Read the model definition and answer for the solid it produces. Units are mm, in the model's axes. Face numbers are marked on the shaded views. A direction names the side the tool comes from. Round coordinates to 2 decimals unless told otherwise and drop trailing zeros. Write each loop counter-clockwise with the first axis right and the second up, starting at its lowest first coordinate (ties: lowest second). Pieces come first, ordered by that corner, then holes. Notation, with made-up numbers: (5.5, 71.5) - (50.5, 71.5) arc R13 cw to (50.5, 85.5) - close; hole circle Ø6 at (39, 0.5). An arc over 180 degrees is marked (long way). Answer as CSV lines item,"result". Start each with the question number.
1) Find section A-A on x = 8.75. Determine the outline of the cut face in (y, z), then the cut area to 3 significant figures.
2) Find section B-B on y = 10. Determine the outline of the cut face in (x, z), then the cut area to 4 significant figures.
3) For a pull along Y with two mould halves and no side action, classify the marked faces 5, 6 and 7 as +Y half, -Y half, draft (parallel to the pull), parting line (faces both ways), or undercut.
4) Consider line 1 along Y through (x, z) = (7.5, 2.75); line 2 along X through (y, z) = (3.75, 7); line 3 along Y through (x, z) = (10, 5). Determine where each line is inside the solid, lowest interval first.
5) Each of these flat-tipped pins is pushed along its axis until it touches: pin 1 (4 mm diameter, centred on x = 15, z = 5, fed in from -Y); pin 2 (1.2 mm diameter, centred on x = 21, y = -1.5, fed in from +Z); pin 3 (0.6 mm diameter, centred on x = 13.5, y = 3.5, fed in from -Z). Where does it stop, or does it pass through?
6) Which of the six approach directions +Z, -Z, +X, -X, +Y, -Y give full straight-line access (tool end or side, diameter ignored) to the marked faces 1, 2, 3 and 4?
from build123d import *

# Parameters (mm, degrees)
BOSS_EXTRUDE1_DEPTH = 7.6
SKETCH2_W           = 17
SKETCH2_H           = 8.9
BOSS_EXTRUDE2_DEPTH = 2
SKETCH3_W           = 20
SKETCH3_H           = 2.43
BOSS_EXTRUDE3_DEPTH = 7.4
SKETCH4_W           = 18
SKETCH4_H           = 2.9
BOSS_EXTRUDE4_DEPTH = 7.67
CUT_EXTRUDE1_DEPTH  = 0.95
SKETCH6_W           = 1.35
SKETCH6_H           = 6.05
CUT_EXTRUDE2_DEPTH  = 0.8
CHAMFER1_SIZE       = 0.5
CHAMFER2_SIZE       = 1
CHAMFER3_SIZE       = 1
SKETCH7_W           = 2.8
SKETCH7_H           = 1.6
BOSS_EXTRUDE5_DEPTH = 2.8
SKETCH8_W           = 2.8
SKETCH8_H           = 0.8
BOSS_EXTRUDE6_DEPTH = 2
CUT_EXTRUDE3_DEPTH  = 30.270462928
CHAMFER4_SIZE       = 0.5
SKETCH10_W          = 2
SKETCH10_H          = 7.95
SKETCH10_W_2        = 1
CUT_EXTRUDE4_DEPTH  = 1
CUT_EXTRUDE5_DEPTH  = 1
SKETCH12_W          = 2
SKETCH12_H          = 1.1
CUT_EXTRUDE6_DEPTH  = 1


with BuildPart() as part:
    # Sketch1 → Boss-Extrude1 (new body)
    with BuildSketch(Plane(origin=(0, 0, 0), x_dir=(1, 0, 0), z_dir=(0, 1, 0))):
        Polygon((0, 0), (0, -11), (22.6, -11), (22.6, 0), (19.8, 0), (19.8, -8.9), (2.8, -8.9), (2.8, 0), align=None)
    extrude(amount=BOSS_EXTRUDE1_DEPTH)

    # Sketch2 → Boss-Extrude2 (add)
    with BuildSketch(Plane(origin=(0, 7.6, 0), x_dir=(1, 0, 0), z_dir=(0, 1, 0))):
        with Locations((11.3, -4.45)):
            Rectangle(SKETCH2_W, SKETCH2_H)
    extrude(amount=-BOSS_EXTRUDE2_DEPTH)

    # Sketch3 → Boss-Extrude3 (add)
    with BuildSketch(Plane(origin=(0, 7.6, 0), x_dir=(1, 0, 0), z_dir=(0, 1, 0))):
        with Locations((11.3, -1.215)):
            Rectangle(SKETCH3_W, SKETCH3_H)
    extrude(amount=BOSS_EXTRUDE3_DEPTH)

    # Sketch4 → Boss-Extrude4 (add)
    with BuildSketch(Plane.XY.offset(2.43)):
        with Locations((11.3, 13.55)):
            Rectangle(SKETCH4_W, SKETCH4_H)
    extrude(amount=BOSS_EXTRUDE4_DEPTH)

    # Sketch5 → Cut-Extrude1 (cut)
    with BuildSketch(Plane(origin=(0, 0, 0), x_dir=(-1, 0, 0), z_dir=(0, 0, -1))):
        Polygon((-19.8, 11.5), (-19.8, 5.6), (-2.8, 5.6), (-2.8, 11.5), (-2.4, 11.5), (-2.4, 15), (-20.2, 15), (-20.2, 11.5), align=None)
    extrude(amount=-CUT_EXTRUDE1_DEPTH, mode=Mode.SUBTRACT)

    # Sketch6 → Cut-Extrude2 (cut)
    with BuildSketch(Plane(origin=(0, 15, 0), x_dir=(1, 0, 0), z_dir=(0, 1, 0))):
        with Locations((3.8, -3.975)):
            Rectangle(SKETCH6_W, SKETCH6_H)
        with Locations((6.3, -3.975)):
            Rectangle(SKETCH6_W, SKETCH6_H)
        with Locations((8.8, -3.975)):
            Rectangle(SKETCH6_W, SKETCH6_H)
        with Locations((11.3, -3.975)):
            Rectangle(SKETCH6_W, SKETCH6_H)
        with Locations((13.8, -3.975)):
            Rectangle(SKETCH6_W, SKETCH6_H)
        with Locations((16.3, -3.975)):
            Rectangle(SKETCH6_W, SKETCH6_H)
        with Locations((18.8, -3.975)):
            Rectangle(SKETCH6_W, SKETCH6_H)
    extrude(amount=-CUT_EXTRUDE2_DEPTH, mode=Mode.SUBTRACT)

    # Chamfer1
    chamfer1_edges = [part.edges().sort_by_distance(p)[0] for p in [
        (20.3, 13.55, 10.1),
        (2.3, 13.55, 10.1),
    ]]
    chamfer(chamfer1_edges, length=CHAMFER1_SIZE)

    # Chamfer2
    chamfer2_edges = [part.edges().sort_by_distance(p)[0] for p in [
        (11.3, 15, 10.1),
    ]]
    chamfer(chamfer2_edges, length=CHAMFER2_SIZE)

    # Chamfer3
    chamfer3_edges = [part.edges().sort_by_distance(p)[0] for p in [
        (11.3, 7.6, 11),
    ]]
    chamfer(chamfer3_edges, length=CHAMFER3_SIZE)

    # Sketch7 → Boss-Extrude5 (add)
    with BuildSketch(Plane.XZ):
        with Locations((1.4, 0.8)):
            Rectangle(SKETCH7_W, SKETCH7_H)
        with Locations((21.2, 0.8)):
            Rectangle(SKETCH7_W, SKETCH7_H)
    extrude(amount=BOSS_EXTRUDE5_DEPTH)

    # Sketch8 → Boss-Extrude6 (add)
    with BuildSketch(Plane(origin=(0, 0, 0), x_dir=(-1, 0, 0), z_dir=(0, 0, -1))):
        with Locations((-21.2, -2.4)):
            Rectangle(SKETCH8_W, SKETCH8_H)
        with Locations((-1.4, -2.4)):
            Rectangle(SKETCH8_W, SKETCH8_H)
    extrude(amount=BOSS_EXTRUDE6_DEPTH)

    # Sketch9 → Cut-Extrude3 (cut, through all)
    with BuildSketch(Plane.ZY):
        with BuildLine():
            ThreePointArc((1.6, 0), (2.1, -0.5), (2.6, 0))
            Line((2.6, 0), (1.6, 0))
        make_face()
        with BuildLine():
            Line((1.6, 0), (2.6, 0))
            ThreePointArc((2.6, 0), (2.1, 0.5), (1.6, 0))
        make_face()
    extrude(amount=-CUT_EXTRUDE3_DEPTH, mode=Mode.SUBTRACT)

    # Chamfer4
    chamfer4_edges = [part.edges().sort_by_distance(p)[0] for p in [
        (1.4, -2.8, 1.6),
        (21.2, -2.8, 1.6),
    ]]
    chamfer(chamfer4_edges, length=CHAMFER4_SIZE)

    # Sketch10 → Cut-Extrude4 (cut)
    with BuildSketch(Plane.XZ.offset(-5.6)):
        with Locations((4.31, 4.925)):
            Rectangle(SKETCH10_W, SKETCH10_H)
        with Locations((6.64, 4.925)):
            Rectangle(SKETCH10_W, SKETCH10_H)
        with Locations((8.97, 4.925)):
            Rectangle(SKETCH10_W, SKETCH10_H)
        with Locations((11.8, 4.925)):
            Rectangle(SKETCH10_W_2, SKETCH10_H)
        with Locations((10.8, 4.925)):
            Rectangle(SKETCH10_W_2, SKETCH10_H)
        with Locations((13.63, 4.925)):
            Rectangle(SKETCH10_W, SKETCH10_H)
        with Locations((15.96, 4.925)):
            Rectangle(SKETCH10_W, SKETCH10_H)
        with Locations((18.29, 4.925)):
            Rectangle(SKETCH10_W, SKETCH10_H)
    extrude(amount=-CUT_EXTRUDE4_DEPTH, mode=Mode.SUBTRACT)

    # Sketch11 → Cut-Extrude5 (cut)
    with BuildSketch(Plane(origin=(0, 0, 8.9), x_dir=(-1, 0, 0), z_dir=(0, 0, -1))):
        Polygon((-19.29, 6.6), (-19.29, 5.6), (-19.29, 0), (-17.29, 0), (-17.29, 5.6), (-17.29, 6.6), align=None)
        Polygon((-16.96, 5.6), (-16.96, 0), (-14.96, 0), (-14.96, 5.6), (-14.96, 6.6), (-16.96, 6.6), align=None)
        Polygon((-14.63, 5.6), (-14.63, 0), (-12.63, 0), (-12.63, 5.6), (-12.63, 6.6), (-14.63, 6.6), align=None)
        Polygon((-12.3, 5.6), (-12.3, 0), (-10.3, 0), (-10.3, 5.6), (-10.3, 6.6), (-12.3, 6.6), align=None)
        Polygon((-9.97, 5.6), (-9.97, 0), (-7.97, 0), (-7.97, 5.6), (-7.97, 6.6), (-9.97, 6.6), align=None)
        Polygon((-7.64, 5.6), (-7.64, 0), (-5.64, 0), (-5.64, 5.6), (-5.64, 6.6), (-7.64, 6.6), align=None)
        Polygon((-5.31, 5.6), (-5.31, 0), (-3.31, 0), (-3.31, 5.6), (-3.31, 6.6), (-5.31, 6.6), align=None)
    extrude(amount=-CUT_EXTRUDE5_DEPTH, mode=Mode.SUBTRACT)

    # Sketch12 → Cut-Extrude6 (cut)
    with BuildSketch(Plane.XZ):
        with Locations((4.31, 10.45)):
            Rectangle(SKETCH12_W, SKETCH12_H)
        with Locations((6.64, 10.45)):
            Rectangle(SKETCH12_W, SKETCH12_H)
        with Locations((8.97, 10.45)):
            Rectangle(SKETCH12_W, SKETCH12_H)
        with Locations((11.3, 10.45)):
            Rectangle(SKETCH12_W, SKETCH12_H)
        with Locations((13.63, 10.45)):
            Rectangle(SKETCH12_W, SKETCH12_H)
        with Locations((15.96, 10.45)):
            Rectangle(SKETCH12_W, SKETCH12_H)
        with Locations((18.29, 10.45)):
            Rectangle(SKETCH12_W, SKETCH12_H)
    extrude(amount=-CUT_EXTRUDE6_DEPTH, mode=Mode.SUBTRACT)


solid = part.part
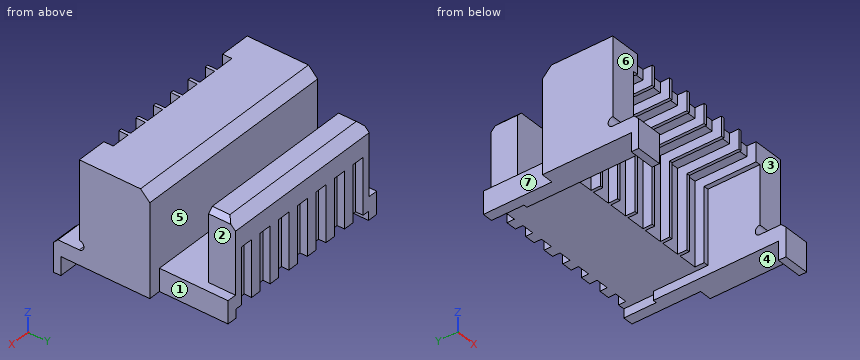
Check values:
1,outline,"(1, 9.9) - (6.6, 9.9) - (6.6, 0.95) - (14.2, 0.95) - (14.2, 7) - (15, 7) - (15, 9.1) - (14, 10.1) - (12.1, 10.1) - (12.1, 2.43) - (7.6, 2.43) - (7.6, 10) - (6.6, 11) - (1, 11) - close"
1,area,"43.6 mm^2"
2,outline,"(1.3, 0) - (2.8, 0) - (2.8, 0.95) - (19.8, 0.95) - (19.8, 0) - (21.3, 0) - (21.3, 2.43) - (1.3, 2.43) - close"
2,area,"32.45 mm^2"
3,face 5,"undercut"
3,face 6,"-Y half"
3,face 7,"draft"
4,line 1,"y = 6.6 to 7.6, 12.1 to 15"
4,line 2,"x = 0 to 2.8, 19.8 to 22.6"
4,line 3,"y = 5.6 to 7.6, 12.1 to 15"
5,pin 1,"stops at y = 5.6"
5,pin 2,"stops at z = 1.6"
5,pin 3,"stops at z = 9.9"
6,face 1,"+Z, -Z, +X, +Y"
6,face 2,"+Z, +X, +Y"
6,face 3,"+Z, +X, -X, -Y"
6,face 4,"-Z, +X, -X, +Y"
